```python
from build123d import *

# Parameters (mm, degrees)
PAD_DEPTH = 45


with BuildPart() as part:
    # Sketch → Pad (new body)
    with BuildSketch(Plane.XY):
        with BuildLine():
            Line((-7.216883, 60.000014), (53.404888, 95.000027))
            Line((53.404888, 95.000027), (55.904888, 90.669901))
            Line((55.904888, 90.669901), (41.155181, 82.154148))
            ThreePointArc((41.155181, 82.154148), (39.32506, 80.324024), (38.655188, 77.824031))
            Line((38.655188, 77.824031), (38.655188, 17.175997))
            ThreePointArc((38.655188, 17.175997), (39.32506, 14.676003), (41.155181, 12.845879))
            Line((41.155181, 12.845879), (55.904888, 4.330126))
            Line((53.404888, 0), (55.904888, 4.330126))
            Line((-7.216883, 35.000014), (53.404888, 0))
            Line((-7.216883, 35.000014), (-14.716886, 22.009634))
            ThreePointArc((-14.716886, 72.990393), (-29.433759, 47.500014), (-14.716886, 22.009634))
            Line((-7.216883, 60.000014), (-14.716886, 72.990393))
        make_face()
        with BuildLine():
            Line((27.603603, 20.66989), (10.283122, 30.669879))
            ThreePointArc((7.783098, 35.000014), (8.45298, 32.500005), (10.283122, 30.669879))
            Line((7.783098, 60.000014), (7.783098, 35.000014))
            ThreePointArc((10.283122, 64.330148), (8.45298, 62.500022), (7.783098, 60.000014))
            Line((10.283122, 64.330148), (27.603603, 74.330137))
            ThreePointArc((35.1036, 70.000014), (32.603599, 74.330136), (27.603603, 74.330137))
            Line((35.1036, 70.000014), (35.1036, 25.000014))
            ThreePointArc((27.603603, 20.66989), (32.603599, 20.669891), (35.1036, 25.000014))
        make_face(mode=Mode.SUBTRACT)
        Polygon((-17.216902, 55.000014), (-2.216902, 55.000014), (-2.216902, 47.500014), (-2.216902, 40.000014), (-17.216902, 40.000014), align=None, mode=Mode.SUBTRACT)
    extrude(amount=PAD_DEPTH)


solid = part.part
```
Input: part model. Units: mm. Frame: model coordinates. A direction names the side the tool comes from. Give positions to 0.01 mm unless a question says otherwise; leave off trailing zeros. Order: outer loops, then holes, each group sorted by start corner. A loop starts at its lowest first (then second) coordinate and runs counter-clockwise, first axis right, second up. Notation, with made-up numbers: M 2.25,68.5 L 34.25,68.5 A7 cw 34.25,77.5 Z; hole C 48,39.5 d2. An arc over 180 degrees is marked long. One line per question, with ' | ' between items. Start each with the question number.
1. First-contact query: pin 1 Ø4.5 at (y, z) = (47.5, 17) entering from +X; pin 2 Ø10 at (x, z) = (44.5, 35) entering from -Y; pin 3 Ø10 at (y, z) = (67, 29.5) entering from -X. Flat tips, straight axial feed; report the tip coordinate or a pass-through.
2. Section query B-B (z = 28). Return the cut outline in (x, y).
3. Pull-direction query (Y, two-part tool) for faces 1 (the face through (-29.43, 47.93, 22.18)), 2 (the face through (18.82, 69.26, 22.18)), 3 (the face through (22.67, 17.745, 22.185)); classes: released by +Y, released by -Y, zero draft, split by the parting line, or undercut.
4. Material intervals for probe 1 along X at (y, z) = (44.5, 19.5); probe 2 along X at (y, z) = (68, 36); probe 3 along Y at (x, z) = (39.5, 30), sorted ascending. Write a range as [from, to].
5. Section query C-C (x = 12). Return the cut outline in (y, z), and give its area (3 significant figures).
6. Access query for faces 4 (the face through (48.63, 86.47, 22.18)), 5 (the face through (-10.91, 28.6, 22.18)), 6 (the face through (7, 48, 45)), 7 (the face through (19.065, 25.6, 22.185)). Directions: +Z, -Z, +X, -X, +Y, -Y. A direction counts if a zero-diameter tool reaches every point of the face in a straight line with its end or side. Return the directions, or none.
7. Section query A-A (x = -6). Return the cut outline in (y, z), and give its area (3 significant figures).
8. Section query D-D (x = 37). Return the cut outline in (y, z), and give its area (3 significant figures).
Here are the results:
1) pin 1: x = 38.66 | pin 2: y = 2.25 | pin 3: x = -25.61
2) outline: M -14.72,22.01 L -7.22,35 L 53.4,0 L 55.9,4.33 L 41.16,12.85 A5 cw 38.66,17.18 L 38.66,77.82 A5 cw 41.16,82.15 L 55.9,90.67 L 53.4,95 L -7.22,60 L -14.72,72.99 A29.43 ccw Z; hole M -17.22,40 L -2.22,40 L -2.22,55 L -17.22,55 Z; hole M 7.78,35 A5 ccw 10.28,30.67 L 27.6,20.67 A5 ccw 35.1,25 L 35.1,70 A5 ccw 27.6,74.33 L 10.28,64.33 A5 ccw 7.78,60 Z
3) face 1: split by the parting line | face 2: undercut | face 3: released by -Y
4) probe 1: [-29.28, -17.22], [-2.22, 7.78], [35.1, 38.66] | probe 2: [-21.12, -11.84], [6.64, 16.64], [35.1, 38.66] | probe 3: [8.03, 14.39], [80.61, 86.97]
5) outline: M 23.91,0 L 29.68,0 L 29.68,45 L 23.91,45 Z; M 65.32,0 L 71.09,0 L 71.09,45 L 65.32,45 Z | area: 520 mm²
6) face 4: +Z, -Z, +X | face 5: +Z, -Z, -Y | face 6: +Z, +X, -X, +Y, -Y | face 7: +Z, -Z
7) outline: M 34.3,0 L 40,0 L 40,45 L 34.3,45 Z; M 55,0 L 60.7,0 L 60.7,45 L 55,45 Z | area: 513 mm²
8) outline: M 9.47,0 L 85.53,0 L 85.53,45 L 9.47,45 Z | area: 3,420 mm²
